```python
from build123d import *

# Parameters (mm, degrees)
RESSALTO_EXTRUS_O1_DEPTH = 5.4
ESBO_O2_R                = 4
RESSALTO_EXTRUS_O2_DEPTH = 50
ESBO_O3_OUTSIDE_W        = 158.404
ESBO_O3_OUTSIDE_H        = 156.44
ESBO_O3_OUTSIDE_R        = 6.35
CORTE_EXTRUS_O1_DEPTH    = 65
CORTE_EXTRUS_O1_TAPER    = 45


with BuildPart() as part:
    # Esboço1 → Ressalto-extrusão1 (new body)
    with BuildSketch(Plane.XY):
        Polygon((3.666174209, -6.35), (7.332348419, 0), (3.666174209, 6.35), (-3.666174209, 6.35), (-7.332348419, 0), (-3.666174209, -6.35), align=None)
    extrude(amount=RESSALTO_EXTRUS_O1_DEPTH)

    # Esboço2 → Ressalto-extrusão2 (add)
    with BuildSketch(Plane.XY.offset(5.4)):
        Circle(ESBO_O2_R)
    extrude(amount=RESSALTO_EXTRUS_O2_DEPTH)

    # Esboço3 outside → Corte-extrusão1 (cut)
    with BuildSketch(Plane(origin=(0, 0, 0), x_dir=(-1, 0, 0), z_dir=(0, 0, -1))):
        Rectangle(ESBO_O3_OUTSIDE_W, ESBO_O3_OUTSIDE_H)
        Circle(ESBO_O3_OUTSIDE_R, mode=Mode.SUBTRACT)
    extrude(amount=-CORTE_EXTRUS_O1_DEPTH, taper=CORTE_EXTRUS_O1_TAPER, mode=Mode.SUBTRACT)


solid = part.part
```
Could you check a few things on this model? Use its own coordinates, in mm. A direction names the side the tool comes from. Coordinates: 2 decimals unless noted, no trailing zeros. Write each loop counter-clockwise with the first axis right and the second up, starting at its lowest first coordinate (ties: lowest second). Pieces come first, ordered by that corner, then holes. Notation, with made-up numbers: (21.5, -17) -> (62.5, -17) arc R20 ccw to (62.5, 21) -> close; hole circle Ø2 at (16, 30.5). An arc over 180 degrees is marked (long way). Write item = value, one per line. Start each with the question number.
(1) I need wall thicknesses on line 1 (Z direction, x = 6, y = 0.5); line 2 (X direction, y = 0.25, z = 51.5); line 3 (Y direction, x = 4, z = 3). Which ranges of each line are inside material? Lowest first, please. Write a range as [from, to].
(2) Will these pins go through, and if not, where does the flat tip stop? pin 1 (1.5 mm diameter, centred on x = -5.5, z = 7.5, fed in from +Y); pin 2 (1.5 mm diameter, centred on x = -5, y = 2, fed in from +Z); pin 3 (2 mm diameter, centred on y = 3.5, z = 42.5, fed in from -X); pin 4 (1 mm diameter, centred on y = 1, z = 19, fed in from +X).
(3) I want a section at A-A (z = 32). Please give me the cut outline in (x, y), plus the area to 3 significant figures.
(4) Which directions (+Z, -Z, +X, -X, +Y, -Y) give clear straight access to the entire face, cutting with the end or side of a thin tool? Please do faces 1 (the face through (-0.867, -3.905, 30.05)), 2 (the face through (0, 0, 55.4)).
Result set:
q1.line_1 = [0, 5.4]
q1.line_2 = [-3.99, 3.99]
q1.line_3 = [-5.77, 5.77]
q2.pin_1 = through
q2.pin_2 = 5.4
q2.pin_3 = -3.12
q2.pin_4 = 3.97
q3.outline = circle Ø8 at (0, 0)
q3.area = 50.3 mm2
q4.face_1 = +Z
q4.face_2 = +Z, +X, -X, +Y, -Y
